Check sheet for the modelled part. Datum: model origin and axes. Units: mm. Face numbers are marked on the shaded views. A direction names the side the tool comes from. Round coordinates to 2 decimals unless told otherwise and drop trailing zeros. Order: outer loops, then holes, each group sorted by start corner. A loop starts at its lowest first (then second) coordinate and runs counter-clockwise, first axis right, second up. Notation, with made-up numbers: (28, 64) -> (80, 64) arc R15 ccw to (80, 83) -> close; hole circle Ø4 at (55.5, 21.25). An arc over 180 degrees is marked (long way). Answer in a Markdown table with one row per item.
```python
from build123d import *

# Parameters (mm, degrees)
CYLINDER165_R     = 2.5
CYLINDER165_DEPTH = 60
CYLINDER161_R     = 2
CYLINDER161_DEPTH = 10
CYLINDER162_R     = 2
CYLINDER162_DEPTH = 10
CYLINDER163_R     = 2
CYLINDER163_DEPTH = 10
CYLINDER164_R     = 2
CYLINDER164_DEPTH = 10
CYLINDER156_R     = 5.5
CYLINDER156_DEPTH = 1
CYLINDER157_R     = 5
CYLINDER157_DEPTH = 5.82
CYLINDER158_R     = 5
CYLINDER158_DEPTH = 5.82
CYLINDER159_R     = 5
CYLINDER159_DEPTH = 5.82
CYLINDER160_R     = 5
CYLINDER160_DEPTH = 5.82
CYLINDER154_R     = 40
CYLINDER154_DEPTH = 4.5
CYLINDER155_R     = 24
CYLINDER155_DEPTH = 7


with BuildPart() as wirecut004:
    # Cylinder165 → Cylinder165 (new body)
    with BuildSketch(Plane(origin=(134, 32.6, 20), x_dir=(1, 0, 0), z_dir=(0, 0, 1))):
        Circle(CYLINDER165_R)
    extrude(amount=CYLINDER165_DEPTH)


with BuildPart() as cylinder161:
    # Cylinder161 → Cylinder161 (new body)
    with BuildSketch(Plane(origin=(0, -21, 0), x_dir=(1, 0, 0), z_dir=(0, 0, 1))):
        Circle(CYLINDER161_R)
    extrude(amount=CYLINDER161_DEPTH)


with BuildPart() as m3heatsetcuts025:
    # Cylinder162 → Cylinder162 (new body)
    with BuildSketch(Plane(origin=(20.5, -21, 0), x_dir=(1, 0, 0), z_dir=(0, 0, 1))):
        Circle(CYLINDER162_R)
    extrude(amount=CYLINDER162_DEPTH)

    # Fusion103: union Cylinder161
    add(cylinder161.part)


with BuildPart() as m3heatsetcuts025_1:
    # Fusion103 placement: moved
    add(m3heatsetcuts025.part.moved(Location((-5, 39, 70))))


with BuildPart() as cylinder163:
    # Cylinder163 → Cylinder163 (new body)
    with BuildSketch(Plane(origin=(0, -21, 0), x_dir=(1, 0, 0), z_dir=(0, 0, 1))):
        Circle(CYLINDER163_R)
    extrude(amount=CYLINDER163_DEPTH)


with BuildPart() as lightmodulecut005:
    # Cylinder164 → Cylinder164 (new body)
    with BuildSketch(Plane(origin=(20.5, -21, 0), x_dir=(1, 0, 0), z_dir=(0, 0, 1))):
        Circle(CYLINDER164_R)
    extrude(amount=CYLINDER164_DEPTH)

    # Fusion104: union Cylinder163
    add(cylinder163.part)


with BuildPart() as lightmodulecut005_1:
    # Fusion104 placement: moved
    add(lightmodulecut005.part.moved(Location((-5, 3, 70))))

    # Fusion102: union m3HeatSetCuts025
    add(m3heatsetcuts025_1.part)


with BuildPart() as lightmodulecut005_2:
    # Fusion102 placement: moved
    add(lightmodulecut005_1.part.moved(Location((128.75, 10, -1))))

    # Fusion105: union WireCut004
    add(wirecut004.part)


with BuildPart() as cylinder156:
    # Cylinder156 → Cylinder156 (new body)
    with BuildSketch(Plane(origin=(134, 32.6, 65), x_dir=(1, 0, 0), z_dir=(0, 0, 1))):
        Circle(CYLINDER156_R)
    extrude(amount=CYLINDER156_DEPTH)


with BuildPart() as cylinder157:
    # Cylinder157 → Cylinder157 (new body)
    with BuildSketch(Plane(origin=(0, -21, 0), x_dir=(1, 0, 0), z_dir=(0, 0, 1))):
        Circle(CYLINDER157_R)
    extrude(amount=CYLINDER157_DEPTH)


with BuildPart() as m3heatsetcuts021:
    # Cylinder158 → Cylinder158 (new body)
    with BuildSketch(Plane(origin=(20.5, -21, 0), x_dir=(1, 0, 0), z_dir=(0, 0, 1))):
        Circle(CYLINDER158_R)
    extrude(amount=CYLINDER158_DEPTH)

    # Fusion097: union Cylinder157
    add(cylinder157.part)


with BuildPart() as m3heatsetcuts021_1:
    # Fusion097 placement: moved
    add(m3heatsetcuts021.part.moved(Location((-5, 39, 70))))


with BuildPart() as cylinder159:
    # Cylinder159 → Cylinder159 (new body)
    with BuildSketch(Plane(origin=(0, -21, 0), x_dir=(1, 0, 0), z_dir=(0, 0, 1))):
        Circle(CYLINDER159_R)
    extrude(amount=CYLINDER159_DEPTH)


with BuildPart() as m3heatsetcuts023:
    # Cylinder160 → Cylinder160 (new body)
    with BuildSketch(Plane(origin=(20.5, -21, 0), x_dir=(1, 0, 0), z_dir=(0, 0, 1))):
        Circle(CYLINDER160_R)
    extrude(amount=CYLINDER160_DEPTH)

    # Fusion098: union Cylinder159
    add(cylinder159.part)


with BuildPart() as m3heatsetcuts023_1:
    # Fusion098 placement: moved
    add(m3heatsetcuts023.part.moved(Location((-5, 3, 70))))

    # Fusion099: union m3HeatSetCuts021
    add(m3heatsetcuts021_1.part)


with BuildPart() as m3heatsetcuts023_2:
    # Fusion099 placement: moved
    add(m3heatsetcuts023_1.part.moved(Location((128.75, 10, -1))))


with BuildPart() as base014:
    # Cylinder154 → Cylinder154 (new body)
    with BuildSketch(Plane(origin=(136, 0, 65), x_dir=(1, 0, 0), z_dir=(0, 0, 1))):
        Circle(CYLINDER154_R)
    extrude(amount=CYLINDER154_DEPTH)


with BuildPart() as basecut003:
    # Cylinder155 → Cylinder155 (new body)
    with BuildSketch(Plane(origin=(5, 0, 74), x_dir=(1, 0, 0), z_dir=(0, 0, 1))):
        Circle(CYLINDER155_R)
    extrude(amount=CYLINDER155_DEPTH)


with BuildPart() as lightmodule009:
    # Sphere005 → Sphere005 (revolve)
    with BuildSketch(Plane(origin=(5, 0, 74), x_dir=(1, 0, 0), z_dir=(0, -1, 0))):
        with BuildLine():
            ThreePointArc((27.5, 0), (27.349352, 2.874533), (26.899059, 5.717571))
            Line((26.899059, 5.717571), (0, 5.717571))
            Line((0, 5.717571), (0, 0))
            Line((0, 0), (27.5, 0))
        make_face()
    revolve(axis=Axis((5, 0, 74), (0, 0, 1)))

    # Cut053: cut baseCut003
    add(basecut003.part, mode=Mode.SUBTRACT)


with BuildPart() as lightmodule009_1:
    # Cut053 placement: moved
    add(lightmodule009.part.moved(Location((131, 0, -5))))

    # Fusion100: union base014
    add(base014.part)


with BuildPart() as lightmodule009_2:
    # Fusion100 placement: moved
    add(lightmodule009_1.part.moved(Location((-2, 10, 0))))

    # Fusion101: union Cylinder156, m3HeatSetCuts023
    add(cylinder156.part)
    add(m3heatsetcuts023_2.part)

    # Cut054: cut lightModuleCut005
    add(lightmodulecut005_2.part, mode=Mode.SUBTRACT)


with BuildPart() as lightmodule009_3:
    # Cut054 placement: moved
    add(lightmodule009_2.part.moved(Location((-134, -384, -74))))


solid = lightmodule009_3.part
```
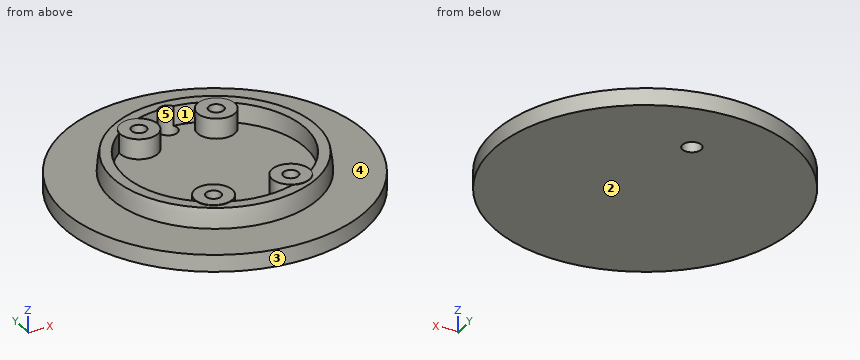
(1) Section check B-B on y = -409. Record the boundary of the cut face in (x, z), plus the area to 3 significant figures.
Solutions:
| item | result |
|---|---|
| outline | (-19.36, -9) -> (19.36, -9) -> (19.36, -4.5) -> (-19.36, -4.5) -> close |
| area | 174 mm^2 |
(2) Depth check by flat-ended pin: pin 1 Ø1.5 at (x, y) = (-8, -399.5) entering from +Z; pin 2 Ø1.5 at (x, z) = (23, -0.5) entering from +Y; pin 3 Ø1.5 at (y, z) = (-400, -2) entering from -X. Enter the tip coordinate at first touch or a pass-through.
Solutions:
| item | result |
|---|---|
| pin 1 | z = 0.72 |
| pin 2 | y = -358.46 |
| pin 3 | x = -10.49 |
(3) Section check D-D on z = -1.5. Give the number of separate pieces and of enclosed holes in the cut face, plus the area to 3 significant figures.
Solutions:
| item | result |
|---|---|
| separate pieces | 1 |
| enclosed holes | 5 |
| area | 749 mm^2 |
(4) Tool access check on the marked faces 4 and 5. Record the directions out of +Z, -Z, +X, -X, +Y, -Y that give a thin tool (end or side, any length) a straight path to the whole face; none if there is none.
Solutions:
| item | result |
|---|---|
| face 4 | +Z |
| face 5 | +Z, -Z |
(5) Draft check along Y on the marked faces 1, 2 and 3. Enter one of: pulls with the +Y half, pulls with the -Y half, needs draft (parallel to the pull), parting line crosses it, or undercut.
Solutions:
| item | result |
|---|---|
| face 1 | undercut |
| face 2 | needs draft |
| face 3 | parting line crosses it |
(6) Section check C-C on x = -32.5. Record the boundary of the cut face in (y, z).
Solutions:
| item | result |
|---|---|
| outline | (-397.32, -9) -> (-350.68, -9) -> (-350.68, -4.5) -> (-397.32, -4.5) -> close |
(7) Scan lines: probe 1 along Y at (x, z) = (-10.25, -0.95); probe 2 along X at (y, z) = (-356, -1.2); probe 3 along X at (y, z) = (-356, -2.3). Record each from-to range of solid material in increasing order. Write a range as from..to.
Solutions:
| item | result |
|---|---|
| probe 1 | -399.19..-394, -390..-387, -361..-358, -354..-348.81 |
| probe 2 | -20.44..-15.87, -15.25..-12.25, -8.25..-5.25, 5.25..8.25, 12.25..15.25, 15.87..20.44 |
| probe 3 | -20.61..-15.87, -15.25..-12.25, -8.25..-5.25, 5.25..8.25, 12.25..15.25, 15.87..20.61 |
(8) Section check A-A on z = -6. Record the boundary of the cut face in (x, y), plus the area to 3 significant figures.
Solutions:
| item | result |
|---|---|
| outline | circle Ø80 at (0, -374); hole circle Ø5 at (0, -351.4) |
| area | 5,010 mm^2 |
